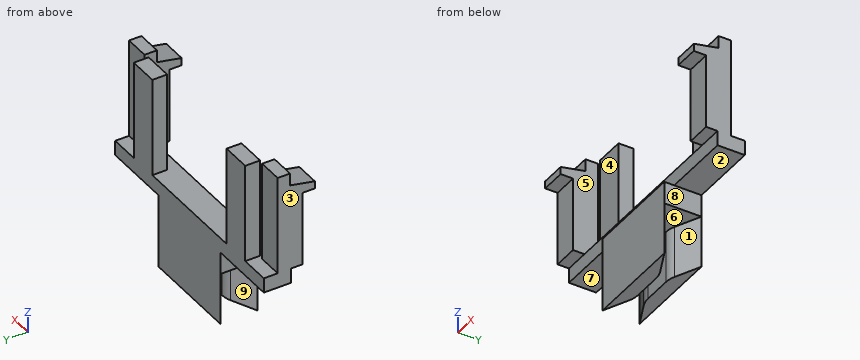
from build123d import *

# Parameters (mm, degrees)
F0_W      = 14
F0_H      = 5.5
F1_DEPTH  = 3
F0_W_2    = 10
F0_H_2    = 2
F2_DEPTH  = 4.5
F4_DEPTH  = 10.5
F5_W      = 6
F5_H      = 3
F5_W_2    = 5
F5_H_2    = 2.7
F5_H_3    = 2.3
F6_DEPTH  = 15
F6_FACE_W = 6
F6_FACE_H = 3
F7_W      = 5
F7_H      = 2.5
F8_DEPTH  = 5
F10_DEPTH = 5
F12_R     = 5


# Not quite as in the source:
# - a feature names something its author has since deleted; it is built from what else it names


with BuildPart() as f1:
    # F0 (on Top) → F1 (new body)
    with BuildSketch(Plane.XY):
        with Locations((17, 0)):
            Rectangle(F0_W, F0_H)
        Polygon((0, -2.75), (10, -2.75), (10, 2.75), (-10, 2.75), (-10, -2.75), align=None)
    extrude(amount=F1_DEPTH)

    # F0 (on Top) → F2 (join)
    with BuildSketch(Plane.XY):
        Polygon((0, -2.75), (10, -2.75), (10, 2.75), (-10, 2.75), (-10, -2.75), align=None)
        with Locations((-5, -3.75)):
            Rectangle(F0_W_2, F0_H_2)
        with Locations((5, -3.75)):
            Rectangle(F0_W_2, F0_H_2)
    extrude(amount=-F2_DEPTH)

    # F3 (on face) → F4 (join)
    with BuildSketch(Plane(origin=(0, 0, -4.5), x_dir=(1, 0, 0), z_dir=(0, 0, -1))):
        Polygon((0, -2.75), (10, -2.75), (4, 0), (0, 0), align=None)
        Polygon((-10, -2.75), (0, -2.75), (0, 0), (-4, 0), align=None)
        Polygon((4, 2), (10, 4.75), (0, 4.75), (0, 2), align=None)
        Polygon((-4, 2), (0, 2), (0, 4.75), (-10, 4.75), align=None)
    extrude(amount=F4_DEPTH)

    # F5 (on face) → F6 (join)
    with BuildSketch(Plane.XY.offset(3)):
        with Locations((15, 1.25)):
            Rectangle(F5_W, F5_H)
        with Locations((21.5, -1.4)):
            Rectangle(F5_W_2, F5_H_2)
        with Locations((21.5, -3.9)):
            Rectangle(F5_W_2, F5_H_3)
    extrude(amount=F6_DEPTH)

    # F6_face (on face) + F7 (on face) → F8 (join)
    with BuildSketch(Plane(origin=(21.5, -2.55, 18), x_dir=(1, 0, 0), z_dir=(0, 0, 1))):
        with Locations((-6.5, 3.8)):
            Rectangle(F6_FACE_W, F6_FACE_H)
    with BuildSketch(Plane.XY.offset(18)):
        with Locations((21.5, -1.3)):
            Rectangle(F7_W, F7_H)
    extrude(amount=F8_DEPTH)

    # F9 (on face) → F10 (join)
    with BuildSketch(Plane.YZ.offset(24)):
        Polygon((-5.05, 18), (-2.55, 18), (-2.55, 19.5), (-7.55, 19.5), (-7.55, 18), align=None)
        Polygon((-7.55, 19.5), (-2.55, 19.5), (-2.55, 20.5), align=None)
    extrude(amount=-F10_DEPTH)

    # F11: F1 across plane


with BuildPart() as f1_1:
    add(f1.part)
    add(f1.part.mirror(Plane.YZ))

    # F12
    f12_edges = [f1_1.edges().sort_by_distance(p)[0] for p in [
        (-4, -2, -9.75),
        (4, -2, -9.75),
        (4, 0, -9.75),
        (-4, 0, -9.75),
    ]]
    fillet(f12_edges, radius=F12_R)


solid = f1_1.part
Here's how the part is built. I have some questions about the finished solid (model axes, mm). Face numbers are marked on the shaded views. A direction names the side the tool comes from. Coordinates: 2 decimals unless noted, no trailing zeros. Order: outer loops, then holes, each group sorted by start corner. A loop starts at its lowest first (then second) coordinate and runs counter-clockwise, first axis right, second up. Notation, with made-up numbers: (82, 42) - (104, 42) arc R8 ccw to (104, 53) - close; hole circle Ø11 at (80, -19). An arc over 180 degrees is marked (long way). Use CSV: the item, a comma, the result in double quotes. Start each with the question number.
1. For the marked faces 5, 6, 7, 8 and 9, which set-ups out of +Z, -Z, +X, -X, +Y, -Y let a thin tool reach every point of the face, with its end or its side?
2. Please list where these lines run through material, in increasing order: line 1 (X direction, y = -2.75, z = 4); line 2 (Y direction, x = 0, z = -11.5); line 3 (Z direction, x = 11, y = -1.25). Write a range as from..to.
3. Suppose I cut it at A-A on z = 13.5. List the corners of the cut face in (x, y) for me.
4. I'm going to push flat-ended pins straight in: pin 1 (4.5 mm diameter, centred on x = -4, y = 1, fed in from +Z); pin 2 (1 mm diameter, centred on y = -5, z = -5, fed in from -X); pin 3 (3 mm diameter, centred on x = -0.5, z = -10, fed in from -Y); pin 4 (2 mm diameter, centred on x = -4.5, y = -6, fed in from -Z). Where does each tip first touch, or does it pass through?
5. Suppose I cut it at C-C on x = -19.5. List the corners of the cut face in (y, z) for me, then the cut area to 3 significant figures.
6. Suppose I cut it at D-D on y = 1.75. List the corners of the cut face in (x, z) for me.
7. If we mould it in two halves opening along X, with no side actions, what happens to the marked faces 1, 2, 3 and 4? For each: +X half, -X half, draft (parallel to the pull), parting line (faces both ways), or undercut.
8. Suppose I cut it at B-B on z = -8. List the corners of the cut face in (x, y) for me.
Output:
1,face 5,"+Z, +Y, -Y"
1,face 6,"-Z"
1,face 7,"-Z, -X, +Y, -Y"
1,face 8,"-Z, +X, +Y, -Y"
1,face 9,"-Z, -X"
2,line 1,"x = -24..-19, 19..24"
2,line 2,"y = -4.75..-2, 0..2.75"
2,line 3,"z = 0..3"
3,outline,"(-24, -5.05) - (-19, -5.05) - (-19, -0.05) - (-24, -0.05) - close; (-18, -0.25) - (-12, -0.25) - (-12, 2.75) - (-18, 2.75) - close; (12, -0.25) - (18, -0.25) - (18, 2.75) - (12, 2.75) - close; (19, -5.05) - (24, -5.05) - (24, -0.05) - (19, -0.05) - close"
4,pin 1,"stops at z = 3"
4,pin 2,"stops at x = -10"
4,pin 3,"stops at y = -4.75"
4,pin 4,"passes through"
5,outline,"(-7.55, 18) - (-5.05, 18) - (-5.05, 3) - (-2.75, 3) - (-2.75, 0) - (2.75, 0) - (2.75, 3) - (-0.05, 3) - (-0.05, 23) - (-2.55, 23) - (-2.55, 20.5) - (-7.55, 19.5) - close"
5,area,"114 mm2"
6,outline,"(-24, 0) - (-10, 0) - (-10, -4.5) - (-7.82, -4.5) - (-7.82, -15) - (7.82, -15) - (7.82, -4.5) - (10, -4.5) - (10, 0) - (24, 0) - (24, 3) - (18, 3) - (18, 23) - (12, 23) - (12, 3) - (-12, 3) - (-12, 23) - (-18, 23) - (-18, 3) - (-24, 3) - close"
7,face 1,"+X half"
7,face 2,"draft"
7,face 3,"-X half"
7,face 4,"undercut"
8,outline,"(-10, -4.75) - (10, -4.75) - (4.99, -2.45) arc R5 ccw to (2.91, -2) - (-2.91, -2) arc R5 ccw to (-4.99, -2.45) - close; (-10, 2.75) - (-4.99, 0.45) arc R5 ccw to (-2.91, 0) - (2.91, 0) arc R5 ccw to (4.99, 0.45) - (10, 2.75) - close"
